For this review, take the finished solid that the model builds, in its own axes (mm). A direction names the side the tool comes from. Round coordinates to 2 decimals unless told otherwise and drop trailing zeros. Loops run counter-clockwise (first coordinate to the right, second up) from the corner with the lowest first, then second, coordinate; pieces in that order, holes last.
1. Consider section C-C on z = 49. State the section outline as (x, y) points.
2. Consider section B-B on x = 7. State the section outline as (y, z) points, then the cut area to 3 significant figures.
3. Consider section A-A on y = -31. State the section outline as (x, z) points, then the cut area to 3 significant figures.
4. Draft analysis for pull direction Z (two halves, no side actions). For faces 1 (the flat face through (-10, -14, -9)), 2 (the flat face through (18, -2, -26)), 3 (the flat face through (18.55, -31.05, -21.67)), state which applies: released by +Z, released by -Z, zero draft, split by the parting line, or undercut.
5. Consider section D-D on z = -4. State the section outline as (x, y) points, then the cut area to 3 significant figures.
6. Tool access review of faces 4 (the flat face through (-9.47, -8.67, 31.92)), 5 (the flat face through (19, -1, -12)), 6 (the flat face through (3, -46, 1)), 7 (the flat face through (13, -25, 23)), 8 (the flat face through (-9, -6.718, 47)): name each direction out of +Z, -Z, +X, -X, +Y, -Y from which nothing blocks a thin tool from reaching the whole face with its end or side.
7. To check wall thickness, follow line 1 along X through (y, z) = (-28, -15); line 2 along X through (y, z) = (-15, 9.5); line 3 along Y through (x, z) = (-16, 43). State the ranges of each line that lie inside material, in increasing order.
8. Clearance check with flat-ended pins moving along their axes: pin 1 Ø8 at (x, z) = (-5, -7) entering from -Y; pin 2 Ø11 at (y, z) = (-25, -19) entering from +X; pin 3 Ø2 at (x, z) = (17, -16.5) entering from -Y; pin 4 Ø6.5 at (y, z) = (-14, -14.96) entering from +X. State where each tip first meets the part, or that it passes through.
from build123d import *

# Parameters (mm, degrees)
SKETCH1_R               = 7
BOSS_EXTRUDE3_DEPTH     = 22
SKETCH8_R               = 5.5
CUT_EXTRUDE1_DEPTH      = 46
SKETCH10_W              = 34.059077951
SKETCH10_H              = 32.597107019
CUT_EXTRUDE2_DEPTH      = 19
SKETCH19_R              = 41
CUT_EXTRUDE5_DEPTH      = 14
CUT_EXTRUDE5_DEPTH_BACK = 10
SKETCH21_W              = 39.040087977
SKETCH21_H              = 19
CUT_EXTRUDE7_DEPTH      = 19
CUT_EXTRUDE8_DEPTH      = 7


with BuildPart() as part:
    # Sketch1 → Boss-Extrude3 (new body, symmetric)
    with BuildSketch(Plane(origin=(0, 0, 0), x_dir=(0, 0, -1), z_dir=(1, 0, 0))):
        with BuildLine():
            Line((0, 0), (24, 0))
            Line((24, 0), (29, -5))
            Line((29, -5), (29, -24))
            Line((29, -24), (0, -58))
            Line((0, -58), (-5.703019947, -58))
            ThreePointArc((-5.703019947, -58), (-7.775768892, -55.305839554), (-9.519025669, -52.387647562))
            ThreePointArc((-9.519025669, -52.387647562), (-11.35140658, -48.033040831), (-12.452414435, -43.438696342))
            ThreePointArc((-12.452414435, -43.438696342), (-14.440768413, -40.168970146), (-18.158792561, -39.262903161))
            Line((-18.158792561, -39.262903161), (-50, -39.262903161))
            Line((-50, -39.262903161), (-57, -32.262903161))
            Line((-57, -32.262903161), (-57, -13.71762228))
            Line((-57, -13.71762228), (-50, -6.71762228))
            Line((-50, -6.71762228), (-43, -6.71762228))
            Line((-43, -6.71762228), (-20.519163329, -10.681600334))
            ThreePointArc((-20.519163329, -10.681600334), (-8.446624302, -8.823458857), (0, 0))
        make_face()
        with Locations((-43, -25.262903161)):
            Circle(SKETCH1_R, mode=Mode.SUBTRACT)
    extrude(amount=BOSS_EXTRUDE3_DEPTH, both=True)

    # Sketch8 → Cut-Extrude1 (cut)
    with BuildSketch(Plane(origin=(22, 0, 0), x_dir=(0, 0, -1), z_dir=(1, 0, 0))):
        with Locations((14.962850045, -14)):
            Circle(SKETCH8_R)
    extrude(amount=-CUT_EXTRUDE1_DEPTH, mode=Mode.SUBTRACT)

    # Sketch10 → Cut-Extrude2 (cut)
    with BuildSketch(Plane(origin=(22, 0, 0), x_dir=(0, 0, -1), z_dir=(1, 0, 0))):
        with Locations((-40.029538976, -22.964349652)):
            Rectangle(SKETCH10_W, SKETCH10_H)
    extrude(amount=-CUT_EXTRUDE2_DEPTH, mode=Mode.SUBTRACT)

    # Sketch19 → Cut-Extrude5 (cut, two sides)
    with BuildSketch(Plane(origin=(0, 0, 0), x_dir=(0, 0, -1), z_dir=(1, 0, 0))) as cut_extrude5_sk:
        with Locations((29, 3.701873436)):
            Circle(SKETCH19_R)
    extrude(amount=CUT_EXTRUDE5_DEPTH, mode=Mode.SUBTRACT)
    extrude(cut_extrude5_sk.sketch, amount=-CUT_EXTRUDE5_DEPTH_BACK, mode=Mode.SUBTRACT)

    # Sketch21 → Cut-Extrude7 (cut)
    with BuildSketch(Plane(origin=(22, 0, 0), x_dir=(0, 0, -1), z_dir=(1, 0, 0))):
        with Locations((-3.479956011, -48.762903161)):
            Rectangle(SKETCH21_W, SKETCH21_H)
    extrude(amount=-CUT_EXTRUDE7_DEPTH, mode=Mode.SUBTRACT)

    # Sketch22 → Cut-Extrude8 (cut)
    with BuildSketch(Plane(origin=(22, 0, 0), x_dir=(0, 0, -1), z_dir=(1, 0, 0))):
        with BuildLine():
            Line((-16.554750267, -38.262903161), (15.520235364, -38.262903161))
            Line((15.520235364, -38.262903161), (28, -23.631454967))
            Line((28, -23.631454967), (28, -5.414213562))
            Line((28, -5.414213562), (23.585786438, -1))
            Line((23.585786438, -1), (0.625702461, -1))
            ThreePointArc((0.625702461, -1), (-8.270776569, -9.856396305), (-20.692811507, -11.666408087))
            Line((-20.692811507, -11.666408087), (-22, -11.435915487))
            Line((-22, -11.435915487), (-22, -38.262903161))
            Line((-22, -38.262903161), (-18.232249909, -38.262903161))
            ThreePointArc((-18.232249909, -38.262903161), (-17.393500088, -38.203988815), (-16.554750267, -38.262903161))
        make_face()
    extrude(amount=-CUT_EXTRUDE8_DEPTH, mode=Mode.SUBTRACT)


solid = part.part
Resolved:
1. outline: (-22, -39.26) - (3, -39.26) - (3, -28.87) - (-22, -28.87) - close; (-22, -21.66) - (3, -21.66) - (3, -6.72) - (-22, -6.72) - close
2. outline: (-39.26, -15.98) - (-36, -18.76) arc R41 cw to (-9.47, 9.83) arc R19 cw to (-10.68, 20.52) - (-10.24, 23) - (-39.26, 23) - (-39.26, 18.16) arc R5 cw to (-39.26, 16.63) - close
2. area: 716 mm2
3. outline: (-22, -23.03) - (-10, -23.03) - (-10, -7.16) - (14, -7.16) - (14, -23.03) - (22, -23.03) - (22, -21.72) - (15, -21.72) - (15, 22) - (22, 22) - (22, 23) - (3, 23) - (3, 38.99) - (-22, 38.99) - close; (-22, 47.01) - (3, 47.01) - (3, 57) - (-22, 57) - close
3. area: 1,990 mm2
4. face 1: zero draft
4. face 2: released by -Z
4. face 3: undercut
5. outline: (-22, -53.31) - (3, -53.31) - (3, -39.26) - (22, -39.26) - (22, -38.26) - (15, -38.26) - (15, -1) - (22, -1) - (22, 0) - (14, 0) - (14, -28.79) - (-10, -28.79) - (-10, 0) - (-22, 0) - close
5. area: 1,130 mm2
6. face 4: +X, -X, +Y
6. face 5: +X
6. face 6: +Z, -Z, +X, -Y
6. face 7: +Z, +X, +Y, -Y
6. face 8: +Z, +X, -X, +Y
7. line 1: x = -22 to -10, 14 to 15
7. line 2: x = -22 to 15
7. line 3: y = -39.26 to -32.26, -18.26 to -6.72
8. pin 1: stops at y = -54.48
8. pin 2: stops at x = 15
8. pin 3: stops at y = -39.26
8. pin 4: passes through
